from build123d import *

# Parameters (mm, degrees)
F0_W     = 400
F0_H     = 400
F1_DEPTH = 3
F2_W     = 20
F2_H     = 3
F2_W_2   = 3
F2_H_2   = 20
F3_DEPTH = 3
F4_R     = 5
F5_DEPTH = 25
F6_W     = 380
F6_H     = 3
F7_DEPTH = 25


with BuildPart() as f1:
    # F0 (on Top) → F1 (new body)
    with BuildSketch(Plane.XY):
        Rectangle(F0_W, F0_H)
    extrude(amount=F1_DEPTH)

    # F2 (on face) → F3 (join, through all)
    with BuildSketch(Plane.XY.offset(3)):
        with Locations((-180, -201.5)):
            Rectangle(F2_W, F2_H)
        with Locations((-140, -201.5)):
            Rectangle(F2_W, F2_H)
        with Locations((-100, -201.5)):
            Rectangle(F2_W, F2_H)
        with Locations((-60, -201.5)):
            Rectangle(F2_W, F2_H)
        with Locations((-20, -201.5)):
            Rectangle(F2_W, F2_H)
        with Locations((20, -201.5)):
            Rectangle(F2_W, F2_H)
        with Locations((60, -201.5)):
            Rectangle(F2_W, F2_H)
        with Locations((100, -201.5)):
            Rectangle(F2_W, F2_H)
        with Locations((140, -201.5)):
            Rectangle(F2_W, F2_H)
        with Locations((180, -201.5)):
            Rectangle(F2_W, F2_H)
        with Locations((201.5, 100)):
            Rectangle(F2_W_2, F2_H_2)
        with Locations((201.5, 180)):
            Rectangle(F2_W_2, F2_H_2)
        with Locations((201.5, 20)):
            Rectangle(F2_W_2, F2_H_2)
        with Locations((201.5, 140)):
            Rectangle(F2_W_2, F2_H_2)
        with Locations((201.5, -20)):
            Rectangle(F2_W_2, F2_H_2)
        with Locations((201.5, 60)):
            Rectangle(F2_W_2, F2_H_2)
        with Locations((201.5, -60)):
            Rectangle(F2_W_2, F2_H_2)
        with Locations((201.5, -180)):
            Rectangle(F2_W_2, F2_H_2)
        with Locations((201.5, -140)):
            Rectangle(F2_W_2, F2_H_2)
        with Locations((201.5, -100)):
            Rectangle(F2_W_2, F2_H_2)
        with Locations((-100, 201.5)):
            Rectangle(F2_W, F2_H)
        with Locations((-180, 201.5)):
            Rectangle(F2_W, F2_H)
        with Locations((-20, 201.5)):
            Rectangle(F2_W, F2_H)
        with Locations((-140, 201.5)):
            Rectangle(F2_W, F2_H)
        with Locations((20, 201.5)):
            Rectangle(F2_W, F2_H)
        with Locations((-60, 201.5)):
            Rectangle(F2_W, F2_H)
        with Locations((60, 201.5)):
            Rectangle(F2_W, F2_H)
        with Locations((180, 201.5)):
            Rectangle(F2_W, F2_H)
        with Locations((140, 201.5)):
            Rectangle(F2_W, F2_H)
        with Locations((100, 201.5)):
            Rectangle(F2_W, F2_H)
        with Locations((-201.5, -100)):
            Rectangle(F2_W_2, F2_H_2)
        with Locations((-201.5, -180)):
            Rectangle(F2_W_2, F2_H_2)
        with Locations((-201.5, -20)):
            Rectangle(F2_W_2, F2_H_2)
        with Locations((-201.5, -140)):
            Rectangle(F2_W_2, F2_H_2)
        with Locations((-201.5, 20)):
            Rectangle(F2_W_2, F2_H_2)
        with Locations((-201.5, -60)):
            Rectangle(F2_W_2, F2_H_2)
        with Locations((-201.5, 60)):
            Rectangle(F2_W_2, F2_H_2)
        with Locations((-201.5, 180)):
            Rectangle(F2_W_2, F2_H_2)
        with Locations((-201.5, 140)):
            Rectangle(F2_W_2, F2_H_2)
        with Locations((-201.5, 100)):
            Rectangle(F2_W_2, F2_H_2)
    extrude(amount=-F3_DEPTH)

    # F4 (on face) → F5 (cut)
    with BuildSketch(Plane.XY.offset(3)):
        with Locations((150, 0)):
            Circle(F4_R)
    extrude(amount=-F5_DEPTH, mode=Mode.SUBTRACT)

    # F6 (on face) → F7 (cut)
    with BuildSketch(Plane.XY.offset(3)):
        with Locations((0, -201.5)):
            Rectangle(F6_W, F6_H)
    extrude(amount=-F7_DEPTH, mode=Mode.SUBTRACT)


solid = f1.part
Part model, mm, in its own coordinate system. Give positions to 0.01 mm unless a question says otherwise; leave off trailing zeros. Loops run counter-clockwise (first coordinate to the right, second up) from the corner with the lowest first, then second, coordinate; pieces in that order, holes last. Notation, with made-up numbers: (69, 13) -> (107, 13) arc R8 cw to (107, 24) -> close; hole circle Ø5 at (-6, 35.5). An arc over 180 degrees is marked (long way). Write each question's results on one line, items separated by ' | '. Start each with the question number.
Q1. Pull direction X, two halves, no side cores. Call faces 1 (the face through (145, 0, 2)), 2 (the face through (-3, 4, 0)): +X half, -X half, draft (parallel to the pull), parting line (faces both ways), or undercut.
Q2. Band-saw the part on A-A on y = 0. List the corners of the cut face in (x, z), plus the area to 3 significant figures.
Q3. Wall check: L1, parallel to Y at x = 81.5, z = 1; L2, parallel to X at y = -4, z = 2.6. Give the ranges that are in metal, low to high.
Q4. Pin check, flat tips, straight feed: P1, Ø0.9, axis at x = -202, z = 2, coming from the +Y side; P2, Ø1.5, axis at x = 202, z = 1, coming from the -Y side; P3, Ø0.9, axis at y = -117.5, z = 1, coming from the +X side. Stop position of each tip, or through.
Results are:
1) face 1: undercut | face 2: draft
2) outline: (-200, 0) -> (145, 0) -> (145, 3) -> (-200, 3) -> close; (155, 0) -> (200, 0) -> (200, 3) -> (155, 3) -> close | area: 1,170 mm²
3) L1: y = -200 to 200 | L2: x = -200 to 147, 153 to 200
4) P1: stops at y = 190 | P2: stops at y = -190 | P3: stops at x = 200
